Could you check a few things on this model? Use its own coordinates, in mm. Face numbers are marked on the shaded views. A direction names the side the tool comes from. Round coordinates to 2 decimals unless told otherwise and drop trailing zeros. Order: outer loops, then holes, each group sorted by start corner. A loop starts at its lowest first (then second) coordinate and runs counter-clockwise, first axis right, second up. Notation, with made-up numbers: (-31, 54.25) - (-10, 54.25) arc R34 ccw to (-10, 85.25) - close; hole circle Ø4 at (17, 74.25). An arc over 180 degrees is marked (long way). Return JSON: item names as keys, results as strings. Group by question number.
from build123d import *

# Parameters (mm, degrees)
F1_DEPTH = 63.5
F2_DEPTH = 25.4
F0_W     = 25.4
F0_H     = 19.05
F4_DEPTH = 25.4
F5_DEPTH = 7.9375
F7_R     = 5.08


# Not quite as in the source:
# - a feature names something its author has since deleted; it is built from what else it names


with BuildPart() as f1:
    # F0 (on Front) → F1 (new body, symmetric)
    with BuildSketch(Plane.XZ):
        Polygon((41.275, -9.525), (41.275, 9.525), (22.225, 9.525), (-41.275, 9.525), (-41.275, -9.525), align=None)
    extrude(amount=F1_DEPTH, both=True)

    # F0 (on Front) → F2 (join, symmetric)
    with BuildSketch(Plane.XZ):
        with BuildLine():
            Line((22.225, 9.525), (41.275, 9.525))
            Line((41.275, 9.525), (41.275, 27.0002))
            ThreePointArc((41.275, 27.0002), (45.9246798487, 38.2255201513), (57.15, 42.8752))
            Line((57.15, 42.8752), (60.325, 42.8752))
            Line((60.325, 42.8752), (60.325, 61.9252))
            Line((60.325, 61.9252), (57.15, 61.9252))
            ThreePointArc((57.15, 61.9252), (55.7573840511, 61.8974240417), (54.3669832056, 61.8141403475))
            add(Edge.make_bspline(
                [(51.6315731061, 61.4864666813), (52.5431025701, 61.5959254015), (53.4550436694, 61.7050265498), (54.3669832056, 61.8141403475)],
                knots=[0.9798743177, 0.9798743177, 0.9798743177, 0.9798743177, 1, 1, 1, 1], degree=3))
            ThreePointArc((51.6315731061, 61.4864666813), (30.5747607323, 49.6610094045), (22.225, 27.0002))
            Line((22.225, 27.0002), (22.225, 9.525))
        make_face()
    extrude(amount=F2_DEPTH, both=True)

    # F0 (on Front) → F4 (join, symmetric)
    with BuildSketch(Plane.XZ):
        with Locations((73.025, 52.4002)):
            Rectangle(F0_W, F0_H)
    extrude(amount=F4_DEPTH, both=True)

    # F0 (on Front) → F5 (join, symmetric)
    with BuildSketch(Plane.XZ):
        with BuildLine():
            Line((-41.275, 9.525), (22.225, 9.525))
            Line((22.225, 9.525), (22.225, 27.0002))
            ThreePointArc((22.225, 27.0002), (30.5747607323, 49.6610094045), (51.6315731061, 61.4864666813))
            add(Edge.make_bspline(
                [(-41.275, 9.525), (-33.3226171476, 23.2066083148), (-16.1059236769, 52.8331960278), (27.7493063598, 58.6186248213), (51.6315731061, 61.4864666813)],
                knots=[0, 0, 0, 0, 0.4525771396, 0.9798743177, 0.9798743177, 0.9798743177, 0.9798743177], degree=3))
        make_face()
    extrude(amount=F5_DEPTH, both=True)

    # F0 (on Front) → F6 (revolve)
    with BuildSketch(Plane.XZ):
        Polygon((85.725, 61.9252), (85.725, 42.8752), (85.725, 38.1), (111.125, 38.1), (111.125, 66.675), (85.725, 66.675), align=None)
    revolve(axis=Axis((85.6968834996, 0, 52.5015871972), (0, 0, -1)))

    # F7
    f7_edges = [f1.edges().sort_by_distance(p)[0] for p in [
        (41.275, -63.5, 0),
        (-41.275, -63.5, 0),
        (41.275, 63.5, 0),
        (-41.275, 63.5, 0),
    ]]
    fillet(f7_edges, radius=F7_R)


solid = f1.part
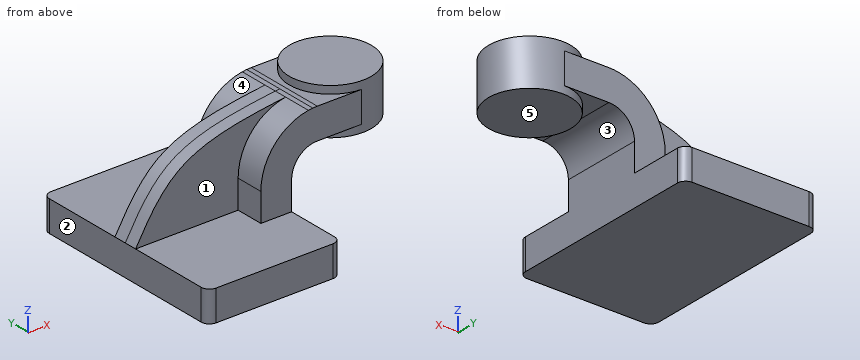
1) We'd pull the mould along X, two halves only. Please class the marked faces 1, 2 and 3: +X half, -X half, draft (parallel to the pull), parting line (faces both ways), or undercut.
2) I want a section at C-C, the plane x = 67. List the corners of the cut face in (y, z) for me (3 decimals), plus the area to 3 significant figures.
3) I want a section at A-A, the plane z = 4. List the corners of the cut face in (x, y) for me (3 decimals), plus the area to 3 significant figures.
4) Will these pins go through, and if not, where does the flat tip stop? pin 1 (1 mm diameter, centred on x = 26.5, y = 22.5, fed in from +Z); pin 2 (8.5 mm diameter, centred on y = 19, z = 16, fed in from -X) (3 decimals); pin 3 (8 mm diameter, centred on x = 27.5, z = 40.5, fed in from +Y).
5) I want a section at B-B, the plane y = 41. List the corners of the cut face in (x, z) for me (3 decimals).
6) For the marked faces 4 and 5, which set-ups out of +Z, -Z, +X, -X, +Y, -Y let a thin tool reach every point of the face, with its end or its side?
7) If I drill on line 1 along X through (y, z) = (11, 24) (3 decimals); line 2 along Z through (x, y) = (-18.5, -26) (3 decimals); line 3 along Z through (x, y) = (70.5, 5) (3 decimals), over which ranges is the centre line in solid material (lowest first)? Write a range as from..to.
Outcome:
{
 "1": {"face 1": "draft", "face 2": "-X half", "face 3": "undercut"},
 "2": {"outline": "(-25.4, 42.875) - (-17.234, 42.875) - (-17.234, 38.1) - (17.234, 38.1) - (17.234, 42.875) - (25.4, 42.875) - (25.4, 61.925) - (17.234, 61.925) - (17.234, 66.675) - (-17.234, 66.675) - (-17.234, 61.925) - (-25.4, 61.925) - close", "area": "1,300 mm^2"},
 "3": {"outline": "(-41.275, -58.42) arc R5.08 ccw to (-36.195, -63.5) - (36.195, -63.5) arc R5.08 ccw to (41.275, -58.42) - (41.275, 58.42) arc R5.08 ccw to (36.195, 63.5) - (-36.195, 63.5) arc R5.08 ccw to (-41.275, 58.42) - close", "area": "10,500 mm^2"},
 "4": {"pin 1": "z = 44.63", "pin 2": "x = 22.225", "pin 3": "y = 25.4"},
 "5": {"outline": "(-41.275, -9.525) - (41.275, -9.525) - (41.275, 9.525) - (-41.275, 9.525) - close"},
 "6": {"face 4": "+Z, -X, +Y", "face 5": "-Z, +X, +Y, -Y"},
 "7": {"line 1": "22.225..41.275", "line 2": "-9.525..9.525", "line 3": "38.1..66.675"}
}
